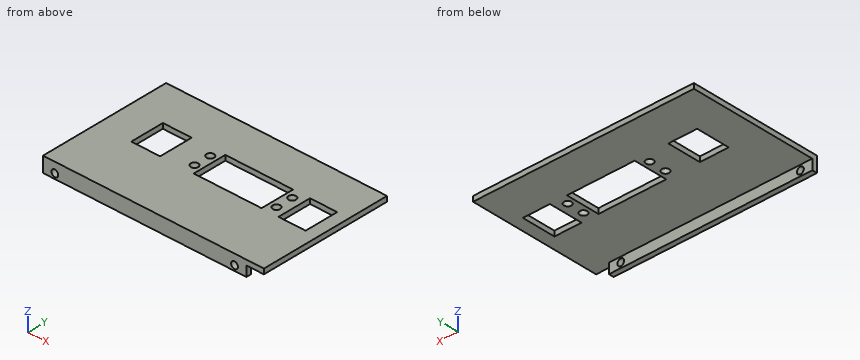
```python
from build123d import *

# Parameters (mm, degrees)
SKETCH_1_W          = 130.339859815
SKETCH_1_H          = 78.03787785
SKETCH_1_R          = 2.2
SKETCH_1_W_2        = 40
SKETCH_1_H_2        = 20
SKETCH_1_W_3        = 17
SKETCH_1_H_3        = 20.000000003
SKETCH_1_W_4        = 16
EXTRUDE_1_DEPTH     = 1.5
SKETCH_2_W          = 120
SKETCH_2_H          = 3
EXTRUDE_2_DEPTH     = 9
SKETCH_3_R          = 2
CUT_EXTRUDE_1_DEPTH = 6


with BuildPart() as part:
    # 草图1 → 凸台-拉伸1 (new, symmetric)
    with BuildSketch(Plane.XY):
        with Locations((26.773633624, -6.330200198)):
            Rectangle(SKETCH_1_W, SKETCH_1_H)
        with Locations((14.641461985, 3.722155933)):
            Circle(SKETCH_1_R, mode=Mode.SUBTRACT)
        with Locations((14.641461985, -6.277844067)):
            Circle(SKETCH_1_R, mode=Mode.SUBTRACT)
        with Locations((63.041461985, 3.722155933)):
            Circle(SKETCH_1_R, mode=Mode.SUBTRACT)
        with Locations((63.041461985, -6.277844067)):
            Circle(SKETCH_1_R, mode=Mode.SUBTRACT)
        with Locations((38.841461985, -1.277844067)):
            Rectangle(SKETCH_1_W_2, SKETCH_1_H_2, mode=Mode.SUBTRACT)
        with Locations((-9.499534143, -1.277844069)):
            Rectangle(SKETCH_1_W_3, SKETCH_1_H_3, mode=Mode.SUBTRACT)
        with Locations((76.841461985, -1.277844067)):
            Rectangle(SKETCH_1_W_4, SKETCH_1_H_2, mode=Mode.SUBTRACT)
    extrude(amount=EXTRUDE_1_DEPTH, both=True)

    # 草图2 → 凸台-拉伸2 (add)
    with BuildSketch(Plane.XY.offset(1.5)):
        with Locations((21.603703717, -43.849139123)):
            Rectangle(SKETCH_2_W, SKETCH_2_H)
    extrude(amount=-EXTRUDE_2_DEPTH)

    # 草图3 → 切除-拉伸1 (cut)
    with BuildSketch(Plane(origin=(0, -42.349139123, 0), x_dir=(1, 0, 0), z_dir=(0, 1, 0))):
        with Locations(Location((-31.396296283, 4.5, 0), (0, 0, 180))):
            Circle(SKETCH_3_R)
        with Locations(Location((74.603703717, 4.5, 0), (0, 0, 180))):
            Circle(SKETCH_3_R)
    extrude(amount=-CUT_EXTRUDE_1_DEPTH, mode=Mode.SUBTRACT)


solid = part.part
```
The model under review builds one solid part; all positions refer to its coordinate system, in mm. Round coordinates to 2 decimals unless told otherwise and drop trailing zeros. Loops run counter-clockwise (first coordinate to the right, second up) from the corner with the lowest first, then second, coordinate; pieces in that order, holes last. Notation, with made-up numbers: (-18.5, 33.5) - (28.5, 33.5) arc R25 cw to (28.5, 56.5) - close; hole circle Ø9 at (69.25, -2.5). An arc over 180 degrees is marked (long way). Use a Markdown table: item, result. Add a question column.
Q1. Add section B-B (x = 70.5). State the section outline as (y, z) points, plus the area to 3 significant figures.
Q2. For probe 1 along Y at (x, z) = (-11.5, 1); probe 2 along X at (y, z) = (4, 0.75); probe 3 along Z at (x, y) = (16, -4), list the stretches that pass through material, from the lowest coordinate up.
Q3. Insertion check: pin 1 Ø5 at (x, z) = (-2.5, -6) entering from +Y; pin 2 Ø2 at (x, y) = (66, -36.5) entering from -Z. Each pin has a flat end and moves straight along its axis. Give the tip position at first contact, or say it passes through.
Q4. Add section A-A (z = -4.5). State the section outline as (x, y) points.
Q5. Add section C-C (x = -22). State the section outline as (y, z) points.
Worked answers:
| question | item | result |
|---|---|---|
| 1 | outline | (-45.35, -7.5) - (-42.35, -7.5) - (-42.35, -1.5) - (-11.28, -1.5) - (-11.28, 1.5) - (-45.35, 1.5) - close; (8.72, -1.5) - (32.69, -1.5) - (32.69, 1.5) - (8.72, 1.5) - close |
| 1 | area | 192 mm² |
| 2 | probe 1 | -45.35 to -11.28, 8.72 to 32.69 |
| 2 | probe 2 | -38.4 to -18, -1 to 12.46, 16.82 to 18.84, 58.84 to 60.86, 65.22 to 68.84, 84.84 to 91.94 |
| 2 | probe 3 | -1.5 to 1.5 |
| 3 | pin 1 | y = -42.35 |
| 3 | pin 2 | z = -1.5 |
| 4 | outline | (-38.4, -45.35) - (-33.4, -45.35) - (-33.4, -42.35) - (-38.4, -42.35) - close; (-29.4, -45.35) - (72.6, -45.35) - (72.6, -42.35) - (-29.4, -42.35) - close; (76.6, -45.35) - (81.6, -45.35) - (81.6, -42.35) - (76.6, -42.35) - close |
| 5 | outline | (-45.35, -7.5) - (-42.35, -7.5) - (-42.35, -1.5) - (32.69, -1.5) - (32.69, 1.5) - (-45.35, 1.5) - close |
